from build123d import *

# Parameters (mm, degrees)
EXTRUDE_1_DEPTH      = 6
EXTRUDE_1_DEPTH_BACK = 2
SKETCH_1_W           = 60
SKETCH_1_H           = 70
SKETCH_1_W_2         = 41
SKETCH_1_H_2         = 51
SKETCH_2_W           = 42
SKETCH_2_H           = 52
CUT_EXTRUDE_2_DEPTH  = 47.486557197
SKETCH_3_W           = 4
SKETCH_3_H           = 3
CHAMFER_2_SIZE       = 3
EXTRUDE_2_DEPTH      = 10
EXTRUDE_3_DEPTH      = 60


with BuildPart() as part:
    # Эскиз1 → Бобышка-Вытянуть1 (new, two sides: drawn at the far end of the back side and taken through both)
    with BuildSketch(Plane.XY.offset(-EXTRUDE_1_DEPTH_BACK)):
        Rectangle(SKETCH_1_W, SKETCH_1_H)
        Rectangle(SKETCH_1_W_2, SKETCH_1_H_2, mode=Mode.SUBTRACT)
    extrude(amount=EXTRUDE_1_DEPTH + EXTRUDE_1_DEPTH_BACK)

    # Эскиз2 → Вырез-Вытянуть2 (cut, through all)
    with BuildSketch(Plane(origin=(0, 0, 0), x_dir=(-1, 0, 0), z_dir=(0, 0, -1))):
        Rectangle(SKETCH_2_W, SKETCH_2_H)
    extrude(amount=-CUT_EXTRUDE_2_DEPTH, mode=Mode.SUBTRACT)

    # Вырез-По траектории1: sweep along a path in Эскиз4
    with BuildLine(Plane(origin=(0, 0, -2), x_dir=(-1, 0, 0), z_dir=(0, 0, -1))) as sweep_1_path:
        Line((-30, 35), (-30, -35))
        Line((-30, -35), (30, -35))
        Line((30, -35), (30, 35))
        Line((30, 35), (-30, 35))
    # Эскиз3 → Вырез-По траектории1 (sweep, cut)
    with BuildSketch(Plane(origin=(0, -35, 0), x_dir=(-1, 0, 0), z_dir=(0, -1, 0))):
        with Locations((-28, 0.5)):
            Rectangle(SKETCH_3_W, SKETCH_3_H)
    sweep(path=sweep_1_path.line, transition=Transition.RIGHT, mode=Mode.SUBTRACT)

    # Фаска2
    chamfer_2_edges = [part.edges().sort_by_distance(p)[0] for p in [
        (26, 0, -2),
        (0, 31, -2),
        (-26, 0, -2),
        (0, -31, -2),
    ]]
    chamfer(chamfer_2_edges, length=CHAMFER_2_SIZE - 0.0001)  # a hair under: the kernel refuses the full size

    # Эскиз5 → Бобышка-Вытянуть2 (add)
    with BuildSketch(Plane(origin=(30, 0, 0), x_dir=(0, 0, -1), z_dir=(1, 0, 0))):
        Polygon((-34.977774789, -27.235428647), (-6, -35), (-6, -29.823619098), (-28.854050432, -23.699894741), align=None)
    extrude_2 = extrude(amount=-EXTRUDE_2_DEPTH)

    # Зеркальное отражение1: Бобышка-Вытянуть2 across plane
    add(extrude_2.mirror(Plane(origin=(0, 0, 0), x_dir=(0, 0, 1), z_dir=(1, 0, 0))))

    # Эскиз6 → Бобышка-Вытянуть3 (add)
    with BuildSketch(Plane(origin=(30, 0, 0), x_dir=(0, 0, -1), z_dir=(1, 0, 0))):
        Polygon((-6, -35), (-1, -36.339745962), (-1, -35), align=None)
    extrude(amount=-EXTRUDE_3_DEPTH)


solid = part.part
Source: CAD feature listing. Evaluate the final solid. Frame: model axes, mm. A direction names the side the tool comes from. Coordinates: 2 decimals unless noted, no trailing zeros. Order: outer loops, then holes, each group sorted by start corner. A loop starts at its lowest first (then second) coordinate and runs counter-clockwise, first axis right, second up. Notation, with made-up numbers: M -7,73 L 13,73 A36 ccw 13,110 Z; hole C 6,34 d8. An arc over 180 degrees is marked long. Write each question's results on one line, items separated by ' | '. Start each with the question number.
Item 1: First-contact query: pin 1 Ø1.6 at (y, z) = (-5.5, -1.5) entering from +X; pin 2 Ø8 at (x, z) = (-3.5, 2) entering from -Y; pin 3 Ø2 at (x, z) = (4.5, -1) entering from -Y. Flat tips, straight axial feed; report the tip coordinate or a pass-through.
Item 2: Cut plane C-C (z = 23). Return loops of the section in (x, y).
Item 3: Line query: probe 1 along X at (y, z) = (-27, 33.5); probe 2 along Y at (x, z) = (-23.5, 0); probe 3 along Z at (x, y) = (-6, 27). Output: solid intervals per line, ascending.
Item 4: Draft query along Y for faces 1 (the face through (0, -29, -1)), 2 (the face through (-25.07, -25.44, 31.87)), 3 (the face through (-20.5, 0, -1)). Return one class per face: pulls with the +Y half, pulls with the -Y half, needs draft (parallel to the pull), parting line crosses it, or undercut.
Item 5: Set-up query: faces 4 (the face through (-27, -9, 1)), 5 (the face through (20, -29, 21)), 6 (the face through (0, 26, 3)), 7 (the face through (-25.07, -26.805, 17.267)). Return all of +Z, -Z, +X, -X, +Y, -Y with unobstructed straight access to the full face (end or side cutting, diameter ignored); none if empty.
Item 6: Cut plane D-D (z = 5). Return loops of the section in (x, y).
Checked values:
1) pin 1: stops at x = 24.3 | pin 2: stops at y = -36.34 | pin 3: stops at y = -30
2) outline: M -30,-30.44 L -20,-30.44 L -20,-25.27 L -30,-25.27 Z; M 20,-30.44 L 30,-30.44 L 30,-25.27 L 20,-25.27 Z
3) probe 1: x = -30 to -20, 20 to 30 | probe 2: y = -30 to 30 | probe 3: z = -2 to 6
4) face 1: pulls with the -Y half | face 2: pulls with the +Y half | face 3: undercut
5) face 4: -Z | face 5: +Z, +Y, -Y | face 6: +Z | face 7: +X, -X, +Y
6) outline: M -30,-35.27 L 30,-35.27 L 30,35 L -30,35 Z; hole M -21,-26 L 21,-26 L 21,26 L -21,26 Z
